from build123d import *

# Parameters (mm, degrees)
SKETCH_1_R          = 2.15
EXTRUDE_1_DEPTH     = 40
SKETCH_3_R          = 1.25
CUT_EXTRUDE_2_DEPTH = 4.000232305
SKETCH_2_W          = 5
SKETCH_2_H          = 10
SKETCH_2_W_2        = 9.8
CUT_EXTRUDE_3_DEPTH = 11
FILLET_1_R          = 1


with BuildPart() as part:
    # 草图1 → 凸台-拉伸1 (new body)
    with BuildSketch(Plane(origin=(0, 0, 0), x_dir=(0, 0, -1), z_dir=(1, 0, 0))):
        with BuildLine():
            Line((-1.96709588, -3.074578638), (-1.665324422, -31.074578638))
            Line((-1.665324422, -31.074578638), (2.334675578, -31.031468429))
            Line((2.334675578, -31.031468429), (2.03290412, -3.031468429))
            ThreePointArc((2.03290412, -3.031468429), (-0.039335781, 3.649788034), (-1.96709588, -3.074578638))
        make_face()
        Circle(SKETCH_1_R, mode=Mode.SUBTRACT)
    extrude(amount=EXTRUDE_1_DEPTH)

    # 草图3 → 切除-拉伸2 (cut)
    with BuildSketch(Plane(origin=(0, 0.021555104, -2), x_dir=(-1, 0, 0), z_dir=(0, 0.010776926175386807, -0.9999419272448828))):
        with Locations(Location((-31.120103863, -27.054826973, 0), (0, 0, 90))):
            Circle(SKETCH_3_R)
        with Locations(Location((-31.120103863, -14.054826973, 0), (0, 0, 90))):
            Circle(SKETCH_3_R)
        with Locations(Location((-9.120103863, -27.054826973, 0), (0, 0, 90))):
            Circle(SKETCH_3_R)
        with Locations(Location((-9.120103863, -14.054826973, 0), (0, 0, 90))):
            Circle(SKETCH_3_R)
    extrude(amount=-CUT_EXTRUDE_2_DEPTH, mode=Mode.SUBTRACT)

    # 草图2 → 切除-拉伸3 (cut, symmetric)
    with BuildSketch(Plane(origin=(0, -0.021555104, 2), x_dir=(1, 0, 0), z_dir=(0, -0.010776926175386815, 0.9999419272448828))):
        with Locations((2.5, -0.278741266)):
            Rectangle(SKETCH_2_W, SKETCH_2_H)
        with Locations((20, -0.278741266)):
            Rectangle(SKETCH_2_W_2, SKETCH_2_H)
        with Locations((37.5, -0.278741266)):
            Rectangle(SKETCH_2_W, SKETCH_2_H)
    extrude(amount=CUT_EXTRUDE_3_DEPTH, both=True, mode=Mode.SUBTRACT)

    # 圆角1
    fillet_1_edges = [part.edges().sort_by_distance(p)[0] for p in [
        (40, -31.053023534, -0.334675578),
        (0, -5.278434715, -0.056888605),
        (0, -31.053023534, -0.334675578),
        (40, -5.278434715, -0.056888605),
    ]]
    fillet(fillet_1_edges, radius=FILLET_1_R)


solid = part.part
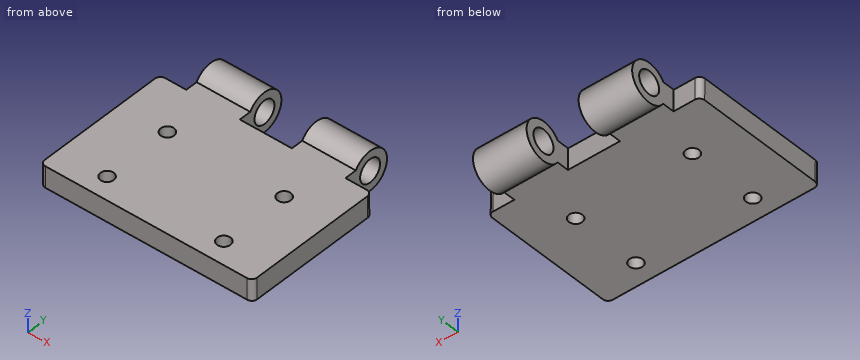
Could you check a few things on this model? Use its own coordinates, in mm. Give positions to 0.01 mm unless a question says otherwise; leave off trailing zeros. Order: outer loops, then holes, each group sorted by start corner. A loop starts at its lowest first (then second) coordinate and runs counter-clockwise, first axis right, second up. Notation, with made-up numbers: (33.25, 61) - (62.25, 61) arc R26 cw to (62.25, 92) - close; hole circle Ø10 at (59.5, 54.5). An arc over 180 degrees is marked (long way). Return JSON: item names as keys, results as strings. Group by question number.
Q1. Suppose I cut it at B-B, the plane z = 2.75. Please give me the cut outline in (x, y), and give its area (3 significant figures).
Q2. Suppose I cut it at D-D, the plane z = -1. State how many separate pieces and enclosed holes the cut face has, and give its area (3 significant figures).
Q3. Suppose I cut it at A-A, the plane y = 0. Please give me the cut outline in (x, z).
Q4. Will these pins go through, and if not, where does the flat tip stop? pin 1 Ø1.5 at (y, z) = (-7, -2.5) entering from -X; pin 2 Ø12 at (x, y) = (10, -11) entering from +Z; pin 3 Ø2 at (y, z) = (-1, 2) entering from +X; pin 4 Ø2 at (x, z) = (8.5, -1.5) entering from +Y.
Q5. Please list where these lines run through material, in increasing order: line 1 along X through (y, z) = (-2.5, -0.5); line 2 along Z through (x, y) = (32.75, 0); line 3 along Y through (x, z) = (22, -2). Write a range as [from, to].
Q6. Suppose I cut it at C-C, the plane x = 6. Please give me the cut outline in (y, z).
Resolved:
{
 "1": {"outline": "(5, -2.4) - (15.1, -2.4) - (15.1, 2.4) - (5, 2.4) - close; (24.9, -2.4) - (35, -2.4) - (35, 2.4) - (24.9, 2.4) - close", "area": "97.0 mm2"},
 "2": {"separate pieces": "3", "enclosed holes": "4", "area": "1,110 mm2"},
 "3": {"outline": "(5, -3.65) - (15.1, -3.65) - (15.1, -2.15) - (5, -2.15) - close; (5, 2.15) - (15.1, 2.15) - (15.1, 3.65) - (5, 3.65) - close; (24.9, -3.65) - (35, -3.65) - (35, -2.15) - (24.9, -2.15) - close; (24.9, 2.15) - (35, 2.15) - (35, 3.65) - (24.9, 3.65) - close"},
 "4": {"pin 1": "stops at x = 0", "pin 2": "stops at z = 1.95", "pin 3": "stops at x = 35", "pin 4": "stops at y = 3.62"},
 "5": {"line 1": "x = [5, 15.1], [24.9, 35]", "line 2": "z = [-3.65, -2.15], [2.15, 3.65]", "line 3": "y = [-31.04, -5.26]"},
 "6": {"outline": "(-31.07, 1.67) - (-31.03, -2.33) - (-3.03, -2.03) arc R3.65 ccw (long way) to (-3.07, 1.97) - close; hole circle Ø4.3 at (0, 0)"}
}
